Part model, mm, in its own coordinate system. A direction names the side the tool comes from. Round coordinates to 2 decimals unless told otherwise and drop trailing zeros. Loops run counter-clockwise (first coordinate to the right, second up) from the corner with the lowest first, then second, coordinate; pieces in that order, holes last.
from build123d import *

# Parameters (mm, degrees)
ESBO_O2_R                  = 5
RESSALTO_EXTRUS_O2_DEPTH   = 12
CORTE_EXTRUS_O1_REACH      = 25.007
CORTE_EXTRUS_O1_END_RADIUS = 5
ESBO_O3_W                  = 4
ESBO_O3_H                  = 2
PADR_OCIRCULAR1_COUNT      = 6


with BuildPart() as part:
    # Esboço2 → Ressalto-extrusão2 (new body)
    with BuildSketch(Plane.XY):
        Polygon((0, 9.814954576), (8.5, 4.907477288), (8.5, -4.907477288), (0, -9.814954576), (-8.5, -4.907477288), (-8.5, 4.907477288), align=None)
        Circle(ESBO_O2_R, mode=Mode.SUBTRACT)
    extrude(amount=RESSALTO_EXTRUS_O2_DEPTH)

    # Corte-extrusão1: up to this cylinder (the profile starts outside it)
    corte_extrus_o1_end = Plane(origin=(0, 0, 10), z_dir=(0, 0, -1)) * Cylinder(CORTE_EXTRUS_O1_END_RADIUS, 61.014, mode=Mode.PRIVATE)
    # Esboço3 → Corte-extrusão1 (cut, up to the surface)
    with BuildSketch(Plane(origin=(8.5, 0, 0), x_dir=(0, 0, -1), z_dir=(1, 0, 0)), mode=Mode.PRIVATE) as corte_extrus_o1_sk1:
        with Locations((-10, 0)):
            Rectangle(ESBO_O3_W, ESBO_O3_H)
    corte_extrus_o1_tool1 = extrude(corte_extrus_o1_sk1.sketch, amount=-CORTE_EXTRUS_O1_REACH, mode=Mode.PRIVATE) - corte_extrus_o1_end
    corte_extrus_o1 = corte_extrus_o1_tool1.solids().sort_by_distance((8.5, 0, 10))[0]
    add(corte_extrus_o1, mode=Mode.SUBTRACT)

    # PadrãoCircular1: Corte-extrusão1 ×6 about axis
    padr_ocircular1_axis = Axis((0, 0, 0), (0, 0, 1))
    for i in range(1, PADR_OCIRCULAR1_COUNT):
        add(corte_extrus_o1.rotate(padr_ocircular1_axis, i * 360 / PADR_OCIRCULAR1_COUNT), mode=Mode.SUBTRACT)


solid = part.part
1) Slice it at B-B, the plane z = 5. Give the cut face in (x, y).
Values:
outline: (-8.5, -4.91) - (0, -9.81) - (8.5, -4.91) - (8.5, 4.91) - (0, 9.81) - (-8.5, 4.91) - close; hole circle Ø10 at (0, 0)
2) Mould opens along X. For faces 1 (the face through (-4.309, 7.327, 5.916)), 2 (the face through (-6, 3, 12)), 3 (the face through (4.228, -5.324, 10.028)) say: released by +X, released by -X, zero draft, split by the parting line, or undercut.
Values:
face 1: released by -X
face 2: zero draft
face 3: undercut
3) Slice it at D-D, the plane y = 4.25. Give the cut face in (x, z).
Values:
outline: (-8.5, 0) - (-2.63, 0) - (-2.63, 8) - (-3.61, 8) - (-3.61, 12) - (-8.5, 12) - close; (2.63, 0) - (8.5, 0) - (8.5, 12) - (3.61, 12) - (3.61, 8) - (2.63, 8) - close
4) Wall check: line 1 along X through (y, z) = (0, 7.5); line 2 along X through (y, z) = (6, 10.5); line 3 along X through (y, z) = (-1.5, 7.5). Give the ranges that are in metal, low to high.
Values:
line 1: x = -8.5 to -5, 5 to 8.5
line 2: x = -6.61 to -4.62, -2.31 to 2.31, 4.62 to 6.61
line 3: x = -8.5 to -4.77, 4.77 to 8.5
5) Tool access for faces 4 (the face through (6, 3, 12)), 5 (the face through (3, -6, 8)), 6 (the face through (7, 1, 10)): list every direction of +Z, -Z, +X, -X, +Y, -Y with a clear straight run to the whole face (end or side of a thin tool).
Values:
face 4: +Z, +X, -X, +Y, -Y
face 5: +Z
face 6: +Z, +X, -X
6) Slice it at A-A, the plane y = 0. Give the cut face in (x, z).
Values:
outline: (-8.5, 0) - (-5, 0) - (-5, 8) - (-8.5, 8) - close; (5, 0) - (8.5, 0) - (8.5, 8) - (5, 8) - close
7) Slice it at C-C, the plane x = -0.25. Give the cut face in (y, z).
Values:
outline: (-9.67, 0) - (-4.99, 0) - (-4.99, 12) - (-9.67, 12) - close; (4.99, 0) - (9.67, 0) - (9.67, 12) - (4.99, 12) - close
8) Drop flat-ended pins along their axis: pin 1 Ø3 at (x, z) = (6.5, 10) entering from +Y; pin 2 Ø4 at (x, y) = (0.5, 1) entering from -Z; pin 3 Ø3 at (x, z) = (6.5, 10.5) entering from -Y; pin 4 Ø0.6 at (x, y) = (7.5, 0.5) entering from +Z. Give the stop position or say it passes through.
Values:
pin 1: stops at y = 6.86
pin 2: passes through
pin 3: stops at y = -6.86
pin 4: stops at z = 8
